from build123d import *

# Parameters (mm, degrees)
SKETCH1_W           = 71.2
SKETCH1_H           = 10
SKETCH1_R           = 2
BOSS_EXTRUDE1_DEPTH = 6
BOSS_EXTRUDE5_START = -6
SKETCH6_W           = 15
SKETCH6_H           = 17
SKETCH6_R           = 2
BOSS_EXTRUDE5_DEPTH = 6
FILLET1_R           = 4
SKETCH7_R           = 2
BOSS_EXTRUDE6_DEPTH = 4.5
FILLET2_R           = 2


with BuildPart() as part:
    # Sketch1 → Boss-Extrude1 (new body)
    with BuildSketch(Plane(origin=(0, 0, 0), x_dir=(1, 0, 0), z_dir=(0, 1, 0))):
        Rectangle(SKETCH1_W, SKETCH1_H)
        with Locations(Location((-32.5, 0, 0), (0, 0, 270))):
            Circle(SKETCH1_R, mode=Mode.SUBTRACT)
        with Locations(Location((-23.7, 0, 0), (0, 0, 270))):
            Circle(SKETCH1_R, mode=Mode.SUBTRACT)
        with Locations(Location((23.7, 0, 0), (0, 0, 270))):
            Circle(SKETCH1_R, mode=Mode.SUBTRACT)
        with Locations(Location((32.5, 0, 0), (0, 0, 270))):
            Circle(SKETCH1_R, mode=Mode.SUBTRACT)
        with Locations(Location((-15, 0, 0), (0, 0, 270))):
            Circle(SKETCH1_R, mode=Mode.SUBTRACT)
        with Locations(Location((15, 0, 0), (0, 0, 270))):
            Circle(SKETCH1_R, mode=Mode.SUBTRACT)
    extrude(amount=BOSS_EXTRUDE1_DEPTH)

    # Sketch6 → Boss-Extrude5 (add)
    # profile 1 of 2: a face of its own
    with BuildSketch(Plane(origin=(0, 6, 0), x_dir=(1, 0, 0), z_dir=(0, 1, 0)).offset(BOSS_EXTRUDE5_START)):
        with Locations((-28.1, 3.5)):
            Rectangle(SKETCH6_W, SKETCH6_H)
        with Locations(Location((-23.7, 0, 0), (0, 0, 270))):
            Circle(SKETCH6_R, mode=Mode.SUBTRACT)
        with Locations(Location((-32.5, 0, 0), (0, 0, 270))):
            Circle(SKETCH6_R, mode=Mode.SUBTRACT)
    # profile 2 of 2: a face of its own
    with BuildSketch(Plane(origin=(0, 6, 0), x_dir=(1, 0, 0), z_dir=(0, 1, 0)).offset(BOSS_EXTRUDE5_START)):
        with Locations((28.1, 3.5)):
            Rectangle(SKETCH6_W, SKETCH6_H)
        with Locations(Location((32.5, 0, 0), (0, 0, 270))):
            Circle(SKETCH6_R, mode=Mode.SUBTRACT)
        with Locations(Location((23.7, 0, 0), (0, 0, 270))):
            Circle(SKETCH6_R, mode=Mode.SUBTRACT)
    extrude(amount=BOSS_EXTRUDE5_DEPTH)

    # Fillet1
    fillet1_edges = [part.edges().sort_by_distance(p)[0] for p in [
        (-20.6, 3, -12),
        (-35.6, 3, -12),
        (35.6, 3, -12),
        (20.6, 3, -12),
    ]]
    fillet(fillet1_edges, radius=FILLET1_R)

    # Sketch7 → Boss-Extrude6 (add)
    # profile 1 of 2: a face of its own
    with BuildSketch(Plane(origin=(0, 6, 0), x_dir=(1, 0, 0), z_dir=(0, 1, 0))):
        with BuildLine():
            Line((31.6, 12), (24.6, 12))
            ThreePointArc((24.6, 12), (21.771572875, 10.828427125), (20.6, 8))
            Line((20.6, 8), (20.6, -5))
            Line((20.6, -5), (35.6, -5))
            Line((35.6, -5), (35.6, 8))
            ThreePointArc((35.6, 8), (34.428427125, 10.828427125), (31.6, 12))
        make_face()
        with Locations(Location((32.5, 0, 0), (0, 0, 270))):
            Circle(SKETCH7_R, mode=Mode.SUBTRACT)
        with Locations(Location((23.7, 0, 0), (0, 0, 270))):
            Circle(SKETCH7_R, mode=Mode.SUBTRACT)
    # profile 2 of 2: a face of its own
    with BuildSketch(Plane(origin=(0, 6, 0), x_dir=(1, 0, 0), z_dir=(0, 1, 0))):
        with BuildLine():
            Line((-24.6, 12), (-31.6, 12))
            ThreePointArc((-31.6, 12), (-34.428427125, 10.828427125), (-35.6, 8))
            Line((-35.6, 8), (-35.6, -5))
            Line((-35.6, -5), (-20.6, -5))
            Line((-20.6, -5), (-20.6, 8))
            ThreePointArc((-20.6, 8), (-21.771572875, 10.828427125), (-24.6, 12))
        make_face()
        with Locations(Location((-23.7, 0, 0), (0, 0, 270))):
            Circle(SKETCH7_R, mode=Mode.SUBTRACT)
        with Locations(Location((-32.5, 0, 0), (0, 0, 270))):
            Circle(SKETCH7_R, mode=Mode.SUBTRACT)
    extrude(amount=BOSS_EXTRUDE6_DEPTH)

    # Fillet2
    fillet2_edges = [part.edges().sort_by_distance(p)[0] for p in [
        (20.6, 8.25, 5),
        (-20.6, 8.25, 5),
        (35.6, 5.25, 5),
        (-35.6, 5.25, 5),
    ]]
    fillet(fillet2_edges, radius=FILLET2_R)


solid = part.part
Check sheet for the modelled part. Datum: model origin and axes. Units: mm. A direction names the side the tool comes from. Give positions to 0.01 mm unless a question says otherwise; leave off trailing zeros. Write each loop counter-clockwise with the first axis right and the second up, starting at its lowest first coordinate (ties: lowest second). Pieces come first, ordered by that corner, then holes. Notation, with made-up numbers: (-22, 89) -> (22, 89) arc R28 ccw to (22, 124) -> close; hole circle Ø1 at (84, -40). An arc over 180 degrees is marked (long way). One line per item, written item: value. Start each with the question number.
Item 1: Section check A-A on z = 0. State how many separate pieces and enclosed holes the cut face has, then the cut area to 3 significant figures.
Item 2: Material ranges on probe 1 along X at (y, z) = (7.5, 0); probe 2 along X at (y, z) = (9, -8.25); probe 3 along Y at (x, z) = (-16, -2.25), recorded low to high. Write a range as from..to.
Item 3: Tool access check on faces 4 (the cylindrical face through (-21.717, 5.176, -0.26)), 5 (the flat face through (0, 3, -5)), 6 (the flat face through (0, 0, -2)), 7 (the cylindrical face through (21.2, 8.28, 4.43)), 8 (the flat face through (20.6, 6.3, -3.8)). Record the directions out of +Z, -Z, +X, -X, +Y, -Y that give a thin tool (end or side, any length) a straight path to the whole face; none if there is none.
Item 4: Draft check along Z on faces 1 (the flat face through (-28, 5, -12)), 2 (the cylindrical face through (21.748, 5.176, -0.434)), 3 (the flat face through (-35.6, 5, -2)). Enter one of: +Z half, -Z half, draft (parallel to the pull), parting line (faces both ways), or undercut.
Item 5: Section check B-B on y = 4.5. Record the cut outline in (x, z).
Item 6: Gauge pin test, flat ends, axial feed: pin 1 (5 mm diameter, centred on x = -15, z = 0, fed in from +Y); pin 2 (2.5 mm diameter, centred on x = 23.7, z = 0, fed in from -Y); pin 3 (4 mm diameter, centred on x = -0.5, y = 1.5, fed in from -Z). Record the tip position at first contact, or that the pin passes through.
Item 7: Section check C-C on x = -15. Record the cut outline in (y, z), then the cut area to 3 significant figures.
Item 8: Section check D-D on z = -4. Record the cut outline in (x, y), then the cut area to 3 significant figures.
Results list:
1. separate pieces: 7
1. enclosed holes: 0
1. area: 346 mm²
2. probe 1: -35.6..-34.5, -30.5..-25.7, -21.7..-20.6, 20.6..21.7, 25.7..30.5, 34.5..35.6
2. probe 2: -35.59..-20.61, 20.61..35.59
2. probe 3: 0..6
3. face 4: +Y, -Y
3. face 5: -Z, +Y, -Y
3. face 6: +Z, -Z, +X, -X, -Y
3. face 7: +Z, +Y
3. face 8: -Z, +Y
4. face 1: -Z half
4. face 2: undercut
4. face 3: draft
5. outline: (-35.6, -8) arc R4 ccw to (-31.6, -12) -> (-24.6, -12) arc R4 ccw to (-20.6, -8) -> (-20.6, -5) -> (20.6, -5) -> (20.6, -8) arc R4 ccw to (24.6, -12) -> (31.6, -12) arc R4 ccw to (35.6, -8) -> (35.6, 3) arc R2 ccw to (33.6, 5) -> (-33.6, 5) arc R2 ccw to (-35.6, 3) -> close; hole circle Ø4 at (-32.5, 0); hole circle Ø4 at (-23.7, 0); hole circle Ø4 at (-15, 0); hole circle Ø4 at (15, 0); hole circle Ø4 at (23.7, 0); hole circle Ø4 at (32.5, 0)
6. pin 1: y = 6
6. pin 2: through
6. pin 3: z = -5
7. outline: (0, -5) -> (6, -5) -> (6, -2) -> (0, -2) -> close; (0, 2) -> (6, 2) -> (6, 5) -> (0, 5) -> close
7. area: 36.0 mm²
8. outline: (-35.6, 0) -> (35.6, 0) -> (35.6, 10.5) -> (20.6, 10.5) -> (20.6, 6) -> (-20.6, 6) -> (-20.6, 10.5) -> (-35.6, 10.5) -> close
8. area: 562 mm²
